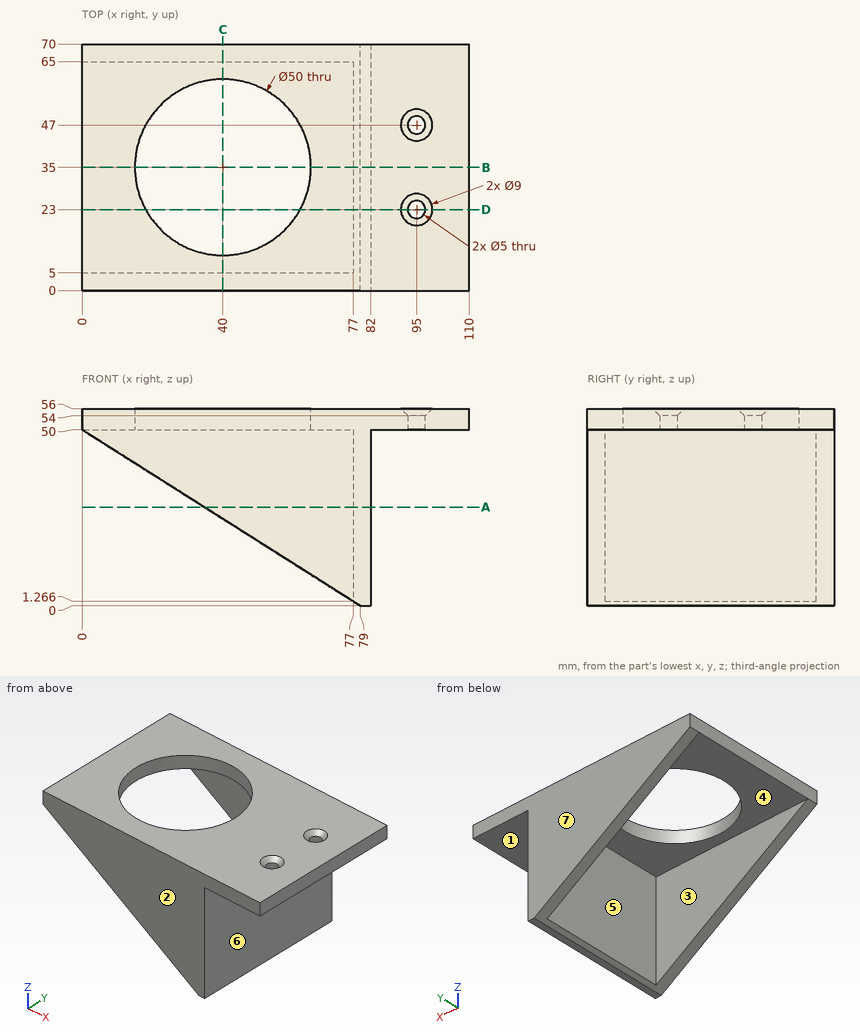
Part print with two shaded views. Sizes in mm from the minimum x, y, z corner. A direction names the side the tool comes from. Coordinates: 2 decimals unless noted, no trailing zeros. Write each loop counter-clockwise with the first axis right and the second up, starting at its lowest first coordinate (ties: lowest second). Pieces come first, ordered by that corner, then holes. Notation, with made-up numbers: M 8.5,64 L 25.5,64 A34 cw 25.5,99 Z; hole C 48.25,34 d8. An arc over 180 degrees is marked long. Return JSON: item names as keys, results as strings.
Item 1: Slice it at D-D, the plane y = 23. Write the cut outline in (x, z).
Findings below:
{"outline": "M 0,50 L 18.07,50 L 18.07,56 L 0,56 Z; M 61.93,50 L 77,50 L 77,1.27 L 79,0 L 82,0 L 82,50 L 92.5,50 L 92.5,54 L 90.5,56 L 61.93,56 Z; M 97.5,50 L 110,50 L 110,56 L 99.5,56 L 97.5,54 Z"}
Item 2: Drop flat-ended pins along their axis: pin 1 Ø4.5 at (x, y) = (95, 23) entering from -Z; pin 2 Ø10 at (y, z) = (34.5, 5.5) entering from +X; pin 3 Ø14 at (x, y) = (98, 36) entering from -Z; pin 4 Ø1.5 at (y, z) = (29.5, 20) entering from -X. Give the stop position or say it passes through.
Findings below:
{"pin 1": "passes through", "pin 2": "stops at x = 82", "pin 3": "stops at z = 50", "pin 4": "stops at x = 77"}
Item 3: Which spindle directions (+Z, -Z, +X, -X, +Y, -Y) get a long thin tool onto all of the face, cutting with end or side? Do the marked faces 1, 2 and 3. Say none if no direction does.
Findings below:
{"face 1": "-Z, +X, +Y, -Y", "face 2": "+Z, -Z, +X, -X, -Y", "face 3": "-Z, -X"}
Item 4: Slice it at C-C, the plane x = 40. Write the cut outline in (y, z).
Findings below:
{"outline": "M 0,24.68 L 5,24.68 L 5,50 L 10,50 L 10,56 L 0,56 Z; M 60,50 L 65,50 L 65,24.68 L 70,24.68 L 70,56 L 60,56 Z"}
Item 5: Two-plate mould, pull along Y, no slides. Class the marked faces 4, 5, 6 and 7: +Y half, -Y half, draft (parallel to the pull), parting line (faces both ways), or undercut.
Findings below:
{"face 4": "undercut", "face 5": "undercut", "face 6": "draft", "face 7": "+Y half"}
Item 6: Slice it at B-B, the plane y = 35. Write the cut outline in (x, z), and give its area (3 significant figures).
Findings below:
{"outline": "M 0,50 L 15,50 L 15,56 L 0,56 Z; M 65,50 L 77,50 L 77,1.27 L 79,0 L 82,0 L 82,50 L 110,50 L 110,56 L 65,56 Z", "area": "609 mm2"}
Item 7: Probe line 1 (Y direction, x = 95, z = 52); line 2 (Y direction, x = 52, z = 38); line 3 (Y direction, x = 40, z = 54.45). List the from-to ranges inside material, lowest first. Write a range as from..to.
Findings below:
{"line 1": "y = 0..20.5, 25.5..44.5, 49.5..70", "line 2": "y = 0..5, 65..70", "line 3": "y = 0..10, 60..70"}
Item 8: Slice it at A-A, the plane z = 28. Write the cut outline in (x, y).
Findings below:
{"outline": "M 34.76,0 L 82,0 L 82,70 L 34.76,70 L 34.76,65 L 77,65 L 77,5 L 34.76,5 Z"}
